from build123d import *

# Parameters (mm, degrees)
EXTRUDE_1_DEPTH = 15
CHAMFER_1_SIZE  = 0.5


with BuildPart() as part:
    # Эскиз1 → Бобышка-Вытянуть1 (new body)
    with BuildSketch(Plane.XY):
        Polygon((2.886751346, 0), (1.443375673, 2.5), (-1.443375673, 2.5), (-2.886751346, 0), (-1.443375673, -2.5), (1.443375673, -2.5), align=None)
    extrude(amount=EXTRUDE_1_DEPTH)

    # Эскиз3 → Вырез-Повернуть1 (revolve, cut)
    with BuildSketch(Plane(origin=(0, 0, 0), x_dir=(1, 0, 0), z_dir=(0, 1, 0))):
        Polygon((-2.886751346, 0), (-1.5, 0), (-1.5, -6), (-2.85, -6), (-2.85, -15), (-2.886751346, -15), align=None)
    revolve(axis=Axis((0, 0, 0), (0, 0, 1)), mode=Mode.SUBTRACT)

    # Фаска1
    chamfer_1_edges = [part.edges().sort_by_distance(p)[0] for p in [
        (1.5, 0, 0),
    ]]
    chamfer(chamfer_1_edges, length=CHAMFER_1_SIZE)

    # Эскиз4 → Отверстие обработанное метчиком M31 (revolve, cut)
    with BuildSketch(Plane(origin=(0, 0, 15), x_dir=(0, -1, 0), z_dir=(1, 0, 0))):
        Polygon((0, 0), (0, 7.751075774), (1.25, 7), (1.25, 5), (1.5, 5), (1.5, 0.105031131), (1.65, 0), align=None)
    revolve(axis=Axis((0, 0, 21.35), (0, 0, -1)), mode=Mode.SUBTRACT)


solid = part.part
Geometry check sheet. Reference: the model listing, model coordinates, mm. A direction names the side the tool comes from. Round coordinates to 2 decimals unless told otherwise and drop trailing zeros. Loops run counter-clockwise (first coordinate to the right, second up) from the corner with the lowest first, then second, coordinate; pieces in that order, holes last. Notation, with made-up numbers: (-18, 54.25) -> (32, 54.25) arc R13 cw to (32, 74.25) -> close; hole circle Ø10 at (-3, 27.5). An arc over 180 degrees is marked (long way). Answer as a JSON object with one key per item and string values. Group by question number.
Item 1: Set-up check for faces 1 (the face through (0, 2, 6)), 2 (the face through (2.155, -1.267, 10.437)), 3 (the face through (1.22, 0.27, 9.01)): record each of +Z, -Z, +X, -X, +Y, -Y from which the full face is reachable in a straight line by a thin tool's end or side.
Item 2: Thickness scan on line 1 along Y through (x, z) = (0, 11.65); line 2 along X through (y, z) = (0, 12.2); line 3 along Z through (x, y) = (1.95, 0.35). Record the ranges inside material, lowest first.
Item 3: Cross-section at A-A, the plane z = 3. Record the cut outline in (x, y), plus the area to 3 significant figures.
Item 4: Depth check by flat-ended pin: pin 1 Ø1.5 at (x, z) = (-1, 5) entering from +Y; pin 2 Ø2.5 at (x, y) = (1, 0.5) entering from -Z; pin 3 Ø1.5 at (x, y) = (-0.5, 0.5) entering from +Z. Enter the tip coordinate at first touch or a pass-through.
Item 5: Cross-section at B-B, the plane y = -2. Record the cut outline in (x, z).
Item 6: Cross-section at C-C, the plane x = -2.5. Record the cut outline in (y, z), plus the area to 3 significant figures.
Item 7: Release check for a two-part mould opening along Y. For faces 4 (the face through (0.21, 0.05, 7.38)), 5 (the face through (-2.175, -1.233, 10.437)), 6 (the face through (1.5, -0.07, 3.29)) record: pulls with the +Y half, pulls with the -Y half, needs draft (parallel to the pull), parting line crosses it, or undercut.
Determined:
{
 "1": {"face 1": "-Z", "face 2": "+Z, -Z, +X, -Y", "face 3": "+Z"},
 "2": {"line 1": "y = -2.5 to -1.5, 1.5 to 2.5", "line 2": "x = -2.85 to -1.5, 1.5 to 2.85", "line 3": "z = 6 to 15"},
 "3": {"outline": "circle Ø3 at (0, 0)", "area": "7.07 mm²"},
 "4": {"pin 1": "stops at y = 1.48", "pin 2": "stops at z = 0", "pin 3": "stops at z = 10"},
 "5": {"outline": "(-1.73, 6) -> (1.73, 6) -> (1.73, 15) -> (-1.73, 15) -> close"},
 "6": {"outline": "(-0.67, 6) -> (0.67, 6) -> (0.67, 15) -> (-0.67, 15) -> close", "area": "12.1 mm²"},
 "7": {"face 4": "undercut", "face 5": "pulls with the -Y half", "face 6": "parting line crosses it"}
}
